Here's how the part is built. I have some questions about the finished solid (model axes, mm). Coordinates: 2 decimals unless noted, no trailing zeros. Write each loop counter-clockwise with the first axis right and the second up, starting at its lowest first coordinate (ties: lowest second). Pieces come first, ordered by that corner, then holes. Notation, with made-up numbers: (60, 23) -> (82, 23) arc R27 ccw to (82, 44) -> close; hole circle Ø5 at (9.5, 86.5). An arc over 180 degrees is marked (long way). Use CSV: the item, a comma, the result in double quotes. Start each with the question number.
```python
from build123d import *

# Parameters (mm, degrees)
F0_R     = 0.762
F1_DEPTH = 3.81


with BuildPart() as f1:
    # F0 (on Top) → F1 (new body)
    with BuildSketch(Plane.XY):
        with BuildLine():
            Line((7.112, 22.352), (-16.002, 22.352))
            ThreePointArc((-16.002, 22.352), (-19.594102, 20.864102), (-21.082, 17.272))
            Line((-21.082, 17.272), (-21.082, -14.732))
            ThreePointArc((-21.082, -14.732), (-19.594102, -18.324102), (-16.002, -19.812))
            Line((-16.002, -19.812), (18.542, -19.812))
            ThreePointArc((18.542, -19.812), (22.134102, -18.324102), (23.622, -14.732))
            Line((23.622, -14.732), (23.622, -3.048))
            ThreePointArc((23.622, -3.048), (22.134102, 0.544102), (18.542, 2.032))
            Line((18.542, 2.032), (17.272, 2.032))
            ThreePointArc((17.272, 2.032), (13.679898, 3.519898), (12.192, 7.112))
            Line((12.192, 7.112), (12.192, 17.272))
            ThreePointArc((12.192, 17.272), (10.704102, 20.864102), (7.112, 22.352))
        make_face()
        with Locations((-17.78, -12.7)):
            Circle(F0_R, mode=Mode.SUBTRACT)
        with Locations((-17.78, -10.16)):
            Circle(F0_R, mode=Mode.SUBTRACT)
        with Locations((-15.24, -12.7)):
            Circle(F0_R, mode=Mode.SUBTRACT)
        with Locations((-12.7, -12.7)):
            Circle(F0_R, mode=Mode.SUBTRACT)
        with Locations((-15.24, -10.16)):
            Circle(F0_R, mode=Mode.SUBTRACT)
        with Locations((-12.7, -10.16)):
            Circle(F0_R, mode=Mode.SUBTRACT)
        with Locations((-7.62, -16.51)):
            Circle(F0_R, mode=Mode.SUBTRACT)
        with Locations((-2.54, -16.51)):
            Circle(F0_R, mode=Mode.SUBTRACT)
        with Locations((0, -16.51)):
            Circle(F0_R, mode=Mode.SUBTRACT)
        with Locations((-7.62, -13.97)):
            Circle(F0_R, mode=Mode.SUBTRACT)
        with Locations((-7.62, -11.43)):
            Circle(F0_R, mode=Mode.SUBTRACT)
        with Locations((-17.78, -2.54)):
            Circle(F0_R, mode=Mode.SUBTRACT)
        with Locations((-15.24, -2.54)):
            Circle(F0_R, mode=Mode.SUBTRACT)
        with Locations((-12.7, -2.54)):
            Circle(F0_R, mode=Mode.SUBTRACT)
        with Locations((-10.16, -2.54)):
            Circle(F0_R, mode=Mode.SUBTRACT)
        with Locations((-7.62, -8.89)):
            Circle(F0_R, mode=Mode.SUBTRACT)
        with Locations((-7.62, -6.35)):
            Circle(F0_R, mode=Mode.SUBTRACT)
        with Locations((-7.62, -3.81)):
            Circle(F0_R, mode=Mode.SUBTRACT)
        with Locations((-7.62, -1.27)):
            Circle(F0_R, mode=Mode.SUBTRACT)
        with Locations((7.62, -16.51)):
            Circle(F0_R, mode=Mode.SUBTRACT)
        with Locations((7.62, -13.97)):
            Circle(F0_R, mode=Mode.SUBTRACT)
        with Locations((7.62, -11.43)):
            Circle(F0_R, mode=Mode.SUBTRACT)
        with Locations((15.24, -12.7)):
            Circle(F0_R, mode=Mode.SUBTRACT)
        with Locations((17.78, -12.7)):
            Circle(F0_R, mode=Mode.SUBTRACT)
        with Locations((15.24, -10.16)):
            Circle(F0_R, mode=Mode.SUBTRACT)
        with Locations((17.78, -10.16)):
            Circle(F0_R, mode=Mode.SUBTRACT)
        with Locations((20.32, -12.7)):
            Circle(F0_R, mode=Mode.SUBTRACT)
        with Locations((20.32, -10.16)):
            Circle(F0_R, mode=Mode.SUBTRACT)
        with Locations((7.62, -8.89)):
            Circle(F0_R, mode=Mode.SUBTRACT)
        with Locations((7.62, -6.35)):
            Circle(F0_R, mode=Mode.SUBTRACT)
        with Locations((7.62, -3.81)):
            Circle(F0_R, mode=Mode.SUBTRACT)
        with Locations((10.16, -2.54)):
            Circle(F0_R, mode=Mode.SUBTRACT)
        with Locations((7.62, -1.27)):
            Circle(F0_R, mode=Mode.SUBTRACT)
        with Locations((12.7, -2.54)):
            Circle(F0_R, mode=Mode.SUBTRACT)
        with Locations((15.24, -2.54)):
            Circle(F0_R, mode=Mode.SUBTRACT)
        with Locations((17.78, -2.54)):
            Circle(F0_R, mode=Mode.SUBTRACT)
        with Locations((-7.62, 1.27)):
            Circle(F0_R, mode=Mode.SUBTRACT)
        with Locations((-7.62, 3.81)):
            Circle(F0_R, mode=Mode.SUBTRACT)
        with Locations((-7.62, 6.35)):
            Circle(F0_R, mode=Mode.SUBTRACT)
        with Locations((-7.62, 8.89)):
            Circle(F0_R, mode=Mode.SUBTRACT)
        with Locations((-7.62, 11.43)):
            Circle(F0_R, mode=Mode.SUBTRACT)
        with Locations((-11.43, 19.05)):
            Circle(F0_R, mode=Mode.SUBTRACT)
        with Locations((-7.62, 13.97)):
            Circle(F0_R, mode=Mode.SUBTRACT)
        with Locations((-7.62, 16.51)):
            Circle(F0_R, mode=Mode.SUBTRACT)
        with Locations((-8.89, 19.05)):
            Circle(F0_R, mode=Mode.SUBTRACT)
        with Locations((-6.35, 19.05)):
            Circle(F0_R, mode=Mode.SUBTRACT)
        with Locations((7.62, 1.27)):
            Circle(F0_R, mode=Mode.SUBTRACT)
        with Locations((7.62, 3.81)):
            Circle(F0_R, mode=Mode.SUBTRACT)
        with Locations((7.62, 6.35)):
            Circle(F0_R, mode=Mode.SUBTRACT)
        with Locations((7.62, 8.89)):
            Circle(F0_R, mode=Mode.SUBTRACT)
        with Locations((7.62, 11.43)):
            Circle(F0_R, mode=Mode.SUBTRACT)
        with Locations((7.62, 13.97)):
            Circle(F0_R, mode=Mode.SUBTRACT)
        with Locations((7.62, 16.51)):
            Circle(F0_R, mode=Mode.SUBTRACT)
    extrude(amount=F1_DEPTH)


solid = f1.part
```
Item 1: I want a section at A-A on y = -11.43. Please give me the cut outline in (x, z).
Item 2: I want a section at B-B on x = -12.7. Please give me the cut outline in (y, z), then the cut area to 3 significant figures.
Item 3: I want a section at C-C on y = 19.05. Please give me the cut outline in (x, z), then the cut area to 3 significant figures.
Item 4: I want a section at D-D on x = 20.32. Please give me the cut outline in (y, z), then the cut area to 3 significant figures.
Item 5: If I drill on line 1 along Y through (x, z) = (17.78, 1.9); line 2 along X through (y, z) = (16.5, 2.35); line 3 along X through (y, z) = (-8.5, 2.35), over which ranges is the centre line in solid material (lowest first)?
Item 6: Thinking about a two-plate mould opening in Y: for faces 1 (the cylindrical face through (-19.633, -18.284, 1.878)), 2 (the cylindrical face through (7.015, 3.346, 1.878)), 3 (the flat face through (-4, 2, 0)), which applies, +Y half, -Y half, draft (parallel to the pull), parting line (faces both ways), or undercut?
Item 7: I'm going to push flat-ended pins straight in: pin 1 (1.4 mm diameter, centred on x = -7.62, y = -6.35, fed in from +Z); pin 2 (1 mm diameter, centred on y = 8.5, z = 3, fed in from +X); pin 3 (1.5 mm diameter, centred on y = 4, z = 1.5, fed in from +X). Where does each tip first touch, or does it pass through?
Geometry says:
1,outline,"(-21.08, 0) -> (-8.38, 0) -> (-8.38, 3.81) -> (-21.08, 3.81) -> close; (-6.86, 0) -> (6.86, 0) -> (6.86, 3.81) -> (-6.86, 3.81) -> close; (8.38, 0) -> (23.62, 0) -> (23.62, 3.81) -> (8.38, 3.81) -> close"
2,outline,"(-19.81, 0) -> (-13.46, 0) -> (-13.46, 3.81) -> (-19.81, 3.81) -> close; (-11.94, 0) -> (-10.92, 0) -> (-10.92, 3.81) -> (-11.94, 3.81) -> close; (-9.4, 0) -> (-3.3, 0) -> (-3.3, 3.81) -> (-9.4, 3.81) -> close; (-1.78, 0) -> (22.35, 0) -> (22.35, 3.81) -> (-1.78, 3.81) -> close"
2,area,"143 mm2"
3,outline,"(-20.76, 0) -> (-12.19, 0) -> (-12.19, 3.81) -> (-20.76, 3.81) -> close; (-10.67, 0) -> (-9.65, 0) -> (-9.65, 3.81) -> (-10.67, 3.81) -> close; (-8.13, 0) -> (-7.11, 0) -> (-7.11, 3.81) -> (-8.13, 3.81) -> close; (-5.59, 0) -> (11.87, 0) -> (11.87, 3.81) -> (-5.59, 3.81) -> close"
3,area,"107 mm2"
4,outline,"(-19.49, 0) -> (-13.46, 0) -> (-13.46, 3.81) -> (-19.49, 3.81) -> close; (-11.94, 0) -> (-10.92, 0) -> (-10.92, 3.81) -> (-11.94, 3.81) -> close; (-9.4, 0) -> (1.71, 0) -> (1.71, 3.81) -> (-9.4, 3.81) -> close"
4,area,"69.2 mm2"
5,line 1,"-19.81 to -13.46, -11.94 to -10.92, -9.4 to -3.3, -1.78 to 2.03"
5,line 2,"-21.08 to -8.38, -6.86 to 6.86, 8.38 to 12.19"
5,line 3,"-21.08 to -8.27, -6.97 to 6.97, 8.27 to 23.62"
6,face 1,"-Y half"
6,face 2,"undercut"
6,face 3,"draft"
7,pin 1,"through"
7,pin 2,"x = 12.19"
7,pin 3,"x = 13.97"
